Geometry: final body of the model. Coordinates: model frame, mm. A direction names the side the tool comes from. Give positions to 0.01 mm unless a question says otherwise; leave off trailing zeros. Order: outer loops, then holes, each group sorted by start corner. A loop starts at its lowest first (then second) coordinate and runs counter-clockwise, first axis right, second up. Notation, with made-up numbers: (-39, -22.75) -> (-11, -22.75) arc R30 ccw to (-11, 3.25) -> close; hole circle Ø1 at (83, 65). An arc over 180 degrees is marked (long way). One line per question, with ' | ' between items.
from build123d import *

# Parameters (mm, degrees)
CHAMFER1_SIZE      = 0.5
SKETCH3_R          = 0.75
CUT_EXTRUDE2_DEPTH = 86.691656537


with BuildPart() as part:
    # Sketch1 → Revolve1 (revolve)
    with BuildSketch(Plane(origin=(0, 0, 0), x_dir=(0, 0, -1), z_dir=(1, 0, 0))):
        Polygon((0, -40.8), (0, 40.8), (3.18, 40.8), (3.18, 19.2), (18.5, 19.2), (18.5, -38.8), (3.18, -38.8), (3.18, -40.8), align=None)
    revolve(axis=Axis((0, -40.8, 0), (0, 1, 0)))

    # Chamfer1
    chamfer1_edges = [part.edges().sort_by_distance(p)[0] for p in [
        (0, 40.8, 3.18),
    ]]
    chamfer(chamfer1_edges, length=CHAMFER1_SIZE)

    # Sketch3 → Cut-Extrude2 (cut, through all)
    with BuildSketch(Plane(origin=(0, 40.8, 0), x_dir=(1, 0, 0), z_dir=(0, 1, 0))):
        with Locations(Location((0, 0, 0), (0, 0, 270))):
            Circle(SKETCH3_R)
    extrude(amount=-CUT_EXTRUDE2_DEPTH, mode=Mode.SUBTRACT)


solid = part.part
1) Material intervals for probe 1 along X at (y, z) = (-3, 0); probe 2 along Y at (x, z) = (-4, 9); probe 3 along Z at (x, y) = (-4.5, -19.5), sorted ascending. Write a range as from..to.
Check result:
probe 1: x = -18.5..-0.75, 0.75..18.5 | probe 2: y = -38.8..19.2 | probe 3: z = -17.94..17.94
2) Pull-direction query (X, two-part tool) for faces 1 (the cylindrical face through (3.1, 29.6, 0.7)), 2 (the flat face through (0, 19.2, 4)), 3 (the cylindrical face through (0.225, 0.571, 0.715)); classes: +X half, -X half, draft (parallel to the pull), parting line (faces both ways), or undercut.
Check result:
face 1: parting line | face 2: draft | face 3: undercut
3) Section A-A on y = 26. Return loops of the section in (x, z).
Check result:
outline: circle Ø6.36 at (0, 0); hole circle Ø1.5 at (0, 0)
4) Contact query for flat-ended pins moving along their axis: pin 1 Ø10 at (y, z) = (8.5, -10) entering from -X; pin 2 Ø8 at (x, z) = (-11, 12) entering from -Y; pin 3 Ø11 at (x, z) = (7, -4.5) entering from +Y; pin 4 Ø2.5 at (x, z) = (0, 0) entering from +Y. Output: stop coordinate, or through.
Check result:
pin 1: stops at x = -17.81 | pin 2: stops at y = -38.8 | pin 3: stops at y = 40.66 | pin 4: stops at y = 40.8
5) Section C-C on y = 2. Return loops of the section in (x, z), plus the area to 3 significant figures.
Check result:
outline: circle Ø37 at (0, 0); hole circle Ø1.5 at (0, 0) | area: 1,070 mm^2
6) Section B-B on z = -8. Return loops of the section in (x, y).
Check result:
outline: (-16.68, -38.8) -> (16.68, -38.8) -> (16.68, 19.2) -> (-16.68, 19.2) -> close
7) Section D-D on x = 10.5. Return loops of the section in (y, z).
Check result:
outline: (-38.8, -15.23) -> (19.2, -15.23) -> (19.2, 15.23) -> (-38.8, 15.23) -> close
8) Set-up query: faces 4 (the cylindrical face through (3.1, -39.8, 0.7)), 5 (the flat face through (-1, -40.8, 0)). Return all of +Z, -Z, +X, -X, +Y, -Y with unobstructed straight access to the full face (end or side cutting, diameter ignored); none if empty.
Check result:
face 4: -Y | face 5: +Z, -Z, +X, -X, -Y
